For this review, use the dimensioned drawing (mm, ordinates from the lowest corner) and the shaded views. A direction names the side the tool comes from. Coordinates: 2 decimals unless noted, no trailing zeros. Loops run counter-clockwise (first coordinate to the right, second up) from the corner with the lowest first, then second, coordinate; pieces in that order, holes last. Notation, with made-up numbers: (70, 68) -> (102, 68) arc R21 cw to (102, 82) -> close; hole circle Ø2 at (12.5, 38). An arc over 180 degrees is marked (long way). Answer as a JSON object with one key per item and string values.
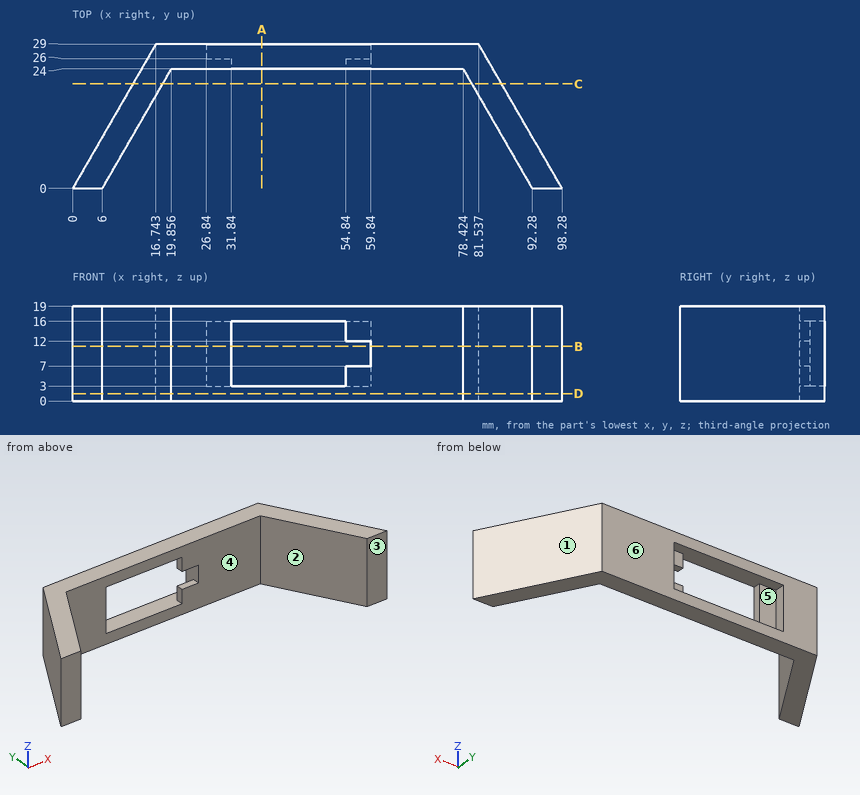
1) Add section B-B, the plane z = 11. Give the boundary of the cut face in (x, y).
Completed:
{"outline": "(0, 0) -> (6, 0) -> (19.86, 24) -> (31.84, 24) -> (31.84, 26) -> (26.84, 26) -> (26.84, 29) -> (16.74, 29) -> close; (59.84, 24) -> (78.42, 24) -> (92.28, 0) -> (98.28, 0) -> (81.54, 29) -> (59.84, 29) -> close"}
2) Clearance check with flat-ended pins moving along their axes: pin 1 Ø4 at (y, z) = (27, 9) entering from -X; pin 2 Ø1.5 at (y, z) = (11.5, 3) entering from +X; pin 3 Ø10 at (x, z) = (33, 4.5) entering from -Y; pin 4 Ø4 at (x, y) = (69, 21) entering from +Z. State where each tip first meets the part, or that it passes through.
Completed:
{"pin 1": "x = 14.43", "pin 2": "x = 92.07", "pin 3": "y = 24", "pin 4": "through"}
3) The part is to be moulded in two halves that separate along X. For the marked faces 1, 2 and 3, say which applies: pulls with the +X half, pulls with the -X half, needs draft (parallel to the pull), parting line crosses it, or undercut.
Completed:
{"face 1": "pulls with the +X half", "face 2": "undercut", "face 3": "needs draft"}
4) Add section A-A, the plane x = 38. Give the boundary of the cut face in (y, z), and give its area (3 significant figures).
Completed:
{"outline": "(24, 0) -> (29, 0) -> (29, 3) -> (24, 3) -> close; (24, 16) -> (29, 16) -> (29, 19) -> (24, 19) -> close", "area": "30.0 mm²"}
5) Wall thickness on probe 1 along Z at (x, y) = (37, 24.5); probe 2 along Y at (x, z) = (21, 4); probe 3 along X at (y, z) = (1.75, 4): over which ranges is each line inside the solid? List them lowest first.
Completed:
{"probe 1": "0 to 3, 16 to 19", "probe 2": "24 to 29", "probe 3": "1.01 to 7.01, 91.27 to 97.27"}
6) Add section C-C, the plane y = 21. Give the boundary of the cut face in (x, z) (1 decimal), and give its area (3 significant figures).
Completed:
{"outline": "(12.1, 0) -> (18.1, 0) -> (18.1, 19) -> (12.1, 19) -> close; (80.2, 0) -> (86.2, 0) -> (86.2, 19) -> (80.2, 19) -> close", "area": "228 mm²"}
7) For the marked faces 4, 5 and 6, list the 3-axis set-ups (+Z, -Z, +X, -X, +Y, -Y) from which the entire face can be reached by the end or side of a thin tool; tool diameter is ignored.
Completed:
{"face 4": "+Z, -Z, -Y", "face 5": "+Y", "face 6": "+Z, -Z, +X, -X, +Y"}
8) Add section D-D, the plane z = 1.5. Give the boundary of the cut face in (x, y).
Completed:
{"outline": "(0, 0) -> (6, 0) -> (19.86, 24) -> (78.42, 24) -> (92.28, 0) -> (98.28, 0) -> (81.54, 29) -> (16.74, 29) -> close"}
